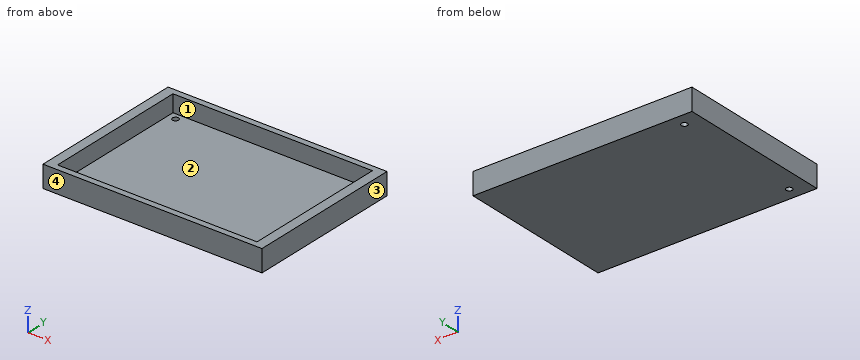
from build123d import *

# Parameters (mm, degrees)
F0_W     = 90
F0_H     = 65
F1_DEPTH = 9
F2_W     = 82
F2_H     = 60
F3_DEPTH = 7
F4_R     = 1.25
F5_DEPTH = 2.001


with BuildPart() as f1:
    # F0 (on Top) → F1 (new body)
    with BuildSketch(Plane.XY):
        with Locations((9.092046, 3.150626)):
            Rectangle(F0_W, F0_H)
    extrude(amount=F1_DEPTH)

    # F2 (on face) → F3 (cut)
    with BuildSketch(Plane.XY.offset(9)):
        with Locations((9.092046, 3.150626)):
            Rectangle(F2_W, F2_H)
    extrude(amount=-F3_DEPTH, mode=Mode.SUBTRACT)

    # F4 (on face) → F5 (cut, through all)
    with BuildSketch(Plane.XY.offset(2)):
        with Locations((-28.657954, 30.400626)):
            Circle(F4_R)
        with Locations((-28.657954, -24.099374)):
            Circle(F4_R)
    extrude(amount=-F5_DEPTH, mode=Mode.SUBTRACT)


solid = f1.part
Design review of the part built by this model. Coordinates are the model's own, in mm. Face numbers are marked on the shaded views. Coordinates: 2 decimals unless noted, no trailing zeros. Write each loop counter-clockwise with the first axis right and the second up, starting at its lowest first coordinate (ties: lowest second). Pieces come first, ordered by that corner, then holes. Notation, with made-up numbers: (36.25, 43) - (72.25, 43) arc R15 ccw to (72.25, 49) - close; hole circle Ø9 at (-32, 22.5). An arc over 180 degrees is marked (long way). One line per item, written item: value.
1) Add section C-C (y = 0). State the section outline as (x, z) points, plus the area to 3 significant figures.
Answer sheet:
outline: (-35.91, 0) - (54.09, 0) - (54.09, 9) - (50.09, 9) - (50.09, 2) - (-31.91, 2) - (-31.91, 9) - (-35.91, 9) - close
area: 236 mm2
2) Insertion check: pin 1 (18 mm diameter, centred on x = -3.5, y = -3, fed in from +Z). The pin has a flat end and moves straight along its axis. Give the tip position at first contact, or say it passes through.
Answer sheet:
pin 1: stops at z = 2
3) Add section A-A (z = 4.5). State the section outline as (x, y) points, plus the area to 3 significant figures.
Answer sheet:
outline: (-35.91, -29.35) - (54.09, -29.35) - (54.09, 35.65) - (-35.91, 35.65) - close; hole (-31.91, -26.85) - (50.09, -26.85) - (50.09, 33.15) - (-31.91, 33.15) - close
area: 930 mm2
4) To check wall thickness, follow probe 1 along X at (y, z) = (23.5, 4.25); probe 2 along Y at (x, z) = (-20, 7); probe 3 along Z at (x, y) = (-16, -20). State the ranges of each line that lie inside material, in increasing order.
Answer sheet:
probe 1: x = -35.91 to -31.91, 50.09 to 54.09
probe 2: y = -29.35 to -26.85, 33.15 to 35.65
probe 3: z = 0 to 2
5) Add section B-B (x = -17). State the section outline as (y, z) points.
Answer sheet:
outline: (-29.35, 0) - (35.65, 0) - (35.65, 9) - (33.15, 9) - (33.15, 2) - (-26.85, 2) - (-26.85, 9) - (-29.35, 9) - close
6) Mouldability with a two-part tool opening along X and no side actions: class the marked faces 1, 2, 3 and 4 as +X half, -X half, draft (parallel to the pull), parting line (faces both ways), or undercut.
Answer sheet:
face 1: undercut
face 2: undercut
face 3: +X half
face 4: draft
